```python
from build123d import *

# Parameters (mm, degrees)
SKETCH1_W              = 50.8
SKETCH1_H              = 19.05
BOSS_EXTRUDE1_DEPTH    = 12.7
SKETCH2_W              = 50.8
SKETCH2_H              = 6.35
BOSS_EXTRUDE2_DEPTH    = 2.2098
F_10_32_TAPPED_HOLE1_D = 4.0386
F_10_32_TAPPED_HOLE2_D = 4.0386


with BuildPart() as part:
    # Sketch1 → Boss-Extrude1 (new body)
    with BuildSketch(Plane(origin=(0, 0, 0), x_dir=(1, 0, 0), z_dir=(0, 1, 0))):
        Rectangle(SKETCH1_W, SKETCH1_H)
    extrude(amount=BOSS_EXTRUDE1_DEPTH)

    # Sketch2 → Boss-Extrude2 (add)
    with BuildSketch(Plane(origin=(0, 12.7, 0), x_dir=(1, 0, 0), z_dir=(0, 1, 0))):
        Rectangle(SKETCH2_W, SKETCH2_H)
    extrude(amount=BOSS_EXTRUDE2_DEPTH)

    # #10-32 Tapped Hole1 (through all)
    with Locations(Plane(origin=(0, 0, -9.525), x_dir=(-1, 0, 0), z_dir=(0, 0, -1))):
        with Locations((12.7, 6.35), (-12.7, 6.35)):
            Hole(F_10_32_TAPPED_HOLE1_D / 2)

    # #10-32 Tapped Hole2 (through all)
    with Locations(Plane(origin=(0, 0, 0), x_dir=(-1, 0, 0), z_dir=(0, -1, 0))):
        with Locations((-19.05, 0), (19.05, 0), (6.35, 0), (-6.35, 0)):
            Hole(F_10_32_TAPPED_HOLE2_D / 2)


solid = part.part
```
Verification items for the finished model (mm, model axes). A direction names the side the tool comes from. Round coordinates to 2 decimals unless told otherwise and drop trailing zeros. Write each loop counter-clockwise with the first axis right and the second up, starting at its lowest first coordinate (ties: lowest second). Pieces come first, ordered by that corner, then holes. Notation, with made-up numbers: (-6, 44.5) -> (33, 44.5) arc R38 ccw to (33, 82.5) -> close; hole circle Ø9 at (32.5, 35). An arc over 180 degrees is marked (long way). Write each question's results on one line, items separated by ' | '. Start each with the question number.
1. Draft check along X on faces 1 (the cylindrical face through (-17.124, 7.559, -0.607)), 2 (the flat face through (0, 12.7, -6)), 3 (the flat face through (-25.4, 7, 0)). Enter one of: +X half, -X half, draft (parallel to the pull), parting line (faces both ways), or undercut.
2. Cross-section at B-B (z = 0). Enter the section's corners in (x, y).
3. Set-up check for faces 4 (the flat face through (0, 0, 0)), 5 (the flat face through (0, 12.7, 6)), 6 (the flat face through (0, 14, -3.175)): record each of +Z, -Z, +X, -X, +Y, -Y from which the full face is reachable in a straight line by a thin tool's end or side.
4. Cross-section at A-A (y = 6.35). Enter the section's corners in (x, z) (3 decimals), then the cut area to 3 significant figures.
5. Material ranges on probe 1 along X at (y, z) = (6.5, 5.5); probe 2 along Z at (x, y) = (-19.05, 5.5) (3 decimals); probe 3 along Y at (x, z) = (-12.5, 4), recorded low to high. Write a range as from..to.
6. Cross-section at D-D (y = 10.5). Enter the section's corners in (x, z) (3 decimals), then the cut area to 4 significant figures.
7. Cross-section at C-C (x = -12.7). Enter the section's corners in (y, z) (3 decimals).
8. Depth check by flat-ended pin: P1, Ø1.1, axis at x = -9, y = 13.5, coming from the -Z side (3 decimals); P2, Ø3, axis at x = -5, z = 7.5, coming from the +Y side; P3, Ø2.5, axis at x = 19.05, z = 0, coming from the +Y side; P4, Ø0.7, axis at x = 12.5, y = 14, coming from the +Z side (3 decimals). Enter the tip coordinate at first touch or a pass-through.
Solutions:
1) face 1: undercut | face 2: draft | face 3: -X half
2) outline: (-25.4, 0) -> (-21.07, 0) -> (-21.07, 14.91) -> (-25.4, 14.91) -> close; (-17.03, 0) -> (-8.37, 0) -> (-8.37, 14.91) -> (-17.03, 14.91) -> close; (-4.33, 0) -> (4.33, 0) -> (4.33, 14.91) -> (-4.33, 14.91) -> close; (8.37, 0) -> (17.03, 0) -> (17.03, 14.91) -> (8.37, 14.91) -> close; (21.07, 0) -> (25.4, 0) -> (25.4, 14.91) -> (21.07, 14.91) -> close; hole circle Ø4.04 at (-12.7, 6.35); hole circle Ø4.04 at (12.7, 6.35)
3) face 4: +Z, -Z, +X, -X, -Y | face 5: +Z, +X, -X, +Y | face 6: -Z, +X, -X, +Y
4) outline: (-25.4, -9.525) -> (-14.719, -9.525) -> (-14.719, 9.525) -> (-25.4, 9.525) -> close; (-10.681, -9.525) -> (10.681, -9.525) -> (10.681, 9.525) -> (-10.681, 9.525) -> close; (14.719, -9.525) -> (25.4, -9.525) -> (25.4, 9.525) -> (14.719, 9.525) -> close; hole circle Ø4.039 at (-19.05, 0); hole circle Ø4.039 at (-6.35, 0); hole circle Ø4.039 at (6.35, 0); hole circle Ø4.039 at (19.05, 0) | area: 763 mm2
5) probe 1: x = -25.4..-14.71, -10.69..10.69, 14.71..25.4 | probe 2: z = -9.525..-2.019, 2.019..9.525 | probe 3: y = 0..4.34, 8.36..12.7
6) outline: (-25.4, -9.525) -> (25.4, -9.525) -> (25.4, 9.525) -> (-25.4, 9.525) -> close; hole circle Ø4.039 at (-19.05, 0); hole circle Ø4.039 at (-6.35, 0); hole circle Ø4.039 at (6.35, 0); hole circle Ø4.039 at (19.05, 0) | area: 916.5 mm2
7) outline: (0, -9.525) -> (4.331, -9.525) -> (4.331, 9.525) -> (0, 9.525) -> close; (8.369, -9.525) -> (12.7, -9.525) -> (12.7, -3.175) -> (14.91, -3.175) -> (14.91, 3.175) -> (12.7, 3.175) -> (12.7, 9.525) -> (8.369, 9.525) -> close
8) P1: stops at z = -3.175 | P2: stops at y = 12.7 | P3: passes through | P4: stops at z = 3.175
